Verification items for the finished model (mm, model axes). Face numbers are marked on the shaded views. Give positions to 0.01 mm unless a question says otherwise; leave off trailing zeros. Order: outer loops, then holes, each group sorted by start corner. A loop starts at its lowest first (then second) coordinate and runs counter-clockwise, first axis right, second up.
from build123d import *

# Parameters (mm, degrees)
F0_W           = 25.4
F0_H           = 31.75
F1_DEPTH       = 25.4
F3_D           = 12.7
F3_CBORE_D     = 15.875
F3_CBORE_DEPTH = 20.32


with BuildPart() as f1:
    # F0 (on Front) → F1 (new body)
    with BuildSketch(Plane.XZ):
        Rectangle(F0_W, F0_H)
    extrude(amount=F1_DEPTH)

    # F3 (through all)
    with Locations(Plane.XY.offset(15.875)):
        with Locations((0, -12.7)):
            CounterBoreHole(F3_D / 2, F3_CBORE_D / 2, F3_CBORE_DEPTH)


solid = f1.part
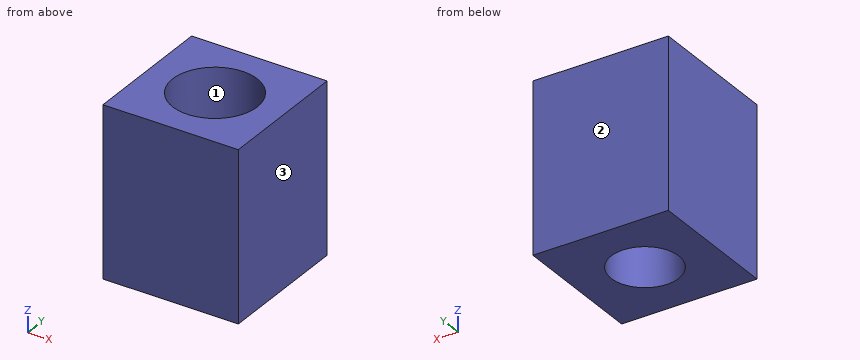
(1) Release check for a two-part mould opening along X. For the marked faces 1, 2 and 3 record: pulls with the +X half, pulls with the -X half, needs draft (parallel to the pull), parting line crosses it, or undercut.
Solved:
face 1: undercut
face 2: needs draft
face 3: pulls with the +X half
(2) Section check D-D, the plane z = 10. Enter the section's corners in (x, y) (1 decimal).
Solved:
outline: (-12.7, -25.4) - (12.7, -25.4) - (12.7, 0) - (-12.7, 0) - close; hole circle Ø15.9 at (0, -12.7)
(3) Scan lines: line 1 (Y direction, x = 0, z = 9.25); line 2 (X direction, y = -13, z = -8); line 3 (Z direction, x = 2, y = -5.75) (3 decimals). Record each from-to range of solid material in increasing order.
Solved:
line 1: y = -25.4 to -20.64, -4.76 to 0
line 2: x = -12.7 to -6.34, 6.34 to 12.7
line 3: z = -15.875 to -4.445
(4) Section check C-C, the plane z = -9. Enter the section's corners in (x, y).
Solved:
outline: (-12.7, -25.4) - (12.7, -25.4) - (12.7, 0) - (-12.7, 0) - close; hole circle Ø12.7 at (0, -12.7)
(5) Go/stop test with a flat-tipped pin: pin 1 (7.5 mm diameter, centred on x = 0, y = -12.7, fed in from -Z). Record where the tip stops, or that it passes through.
Solved:
pin 1: passes through
